Can you work these out from the model? Positions are in its coordinate system, mm. A direction names the side the tool comes from. Round coordinates to 2 decimals unless told otherwise and drop trailing zeros. Order: outer loops, then holes, each group sorted by start corner. A loop starts at its lowest first (then second) coordinate and runs counter-clockwise, first axis right, second up. Notation, with made-up numbers: (-11.5, 86) - (4.5, 86) arc R14 ccw to (4.5, 97) - close; hole circle Ø1 at (54.5, 89). An arc over 180 degrees is marked (long way). Write item = value, one per line.
from build123d import *

# Parameters (mm, degrees)
SKETCH019_W          = 124
SKETCH019_H          = 24.5
SKETCH019_R          = 2.5
PAD010_DEPTH         = 2
SKETCH018_R          = 3.175
PAD011_DEPTH         = 4.1125
PAD012_DEPTH         = 12.25
POCKET005_DEPTH      = 373.382623
POCKET005_DEPTH_BACK = 485.092667
SKETCH022_W          = 3
SKETCH022_H          = 16.275
POCKET006_DEPTH      = 14.161
POCKET006_DEPTH_BACK = 15.001


with BuildPart() as part:
    # Sketch019 → Pad010 (new body)
    with BuildSketch(Plane.XZ.offset(13)):
        with Locations((78, 0)):
            Rectangle(SKETCH019_W, SKETCH019_H)
        with Locations((30, 0)):
            Circle(SKETCH019_R, mode=Mode.SUBTRACT)
        with BuildLine():
            ThreePointArc((90.8685, 2.143), (88.7255, 0), (90.8685, -2.143))
            Line((90.8685, -2.143), (98.806, -2.143))
            ThreePointArc((98.806, -2.143), (100.949, 0), (98.806, 2.143))
            Line((98.806, 2.143), (90.8685, 2.143))
        make_face(mode=Mode.SUBTRACT)
    extrude(amount=PAD010_DEPTH)

    # Sketch018 → Pad011 (join)
    with BuildSketch(Plane.XY.offset(12.25)):
        with BuildLine():
            Line((16, -13), (10.43, -13))
            Line((10.43, -13), (10.43, 3.73))
            ThreePointArc((10.43, 3.73), (2.257465, 13.912767), (-9.45279, 8.137908))
            ThreePointArc((-26.289956, 7.402782), (-17.64833, 2.661824), (-9.45279, 8.137908))
            Line((-26.289956, 7.402782), (-13.355703, -15))
            Line((-13.355703, -15), (16, -15))
            Line((16, -15), (16, -13))
        make_face()
        with Locations((0, 3.73)):
            Circle(SKETCH018_R, mode=Mode.SUBTRACT)
    pad011 = extrude(amount=-PAD011_DEPTH)

    # Mirrored003: Pad011 across XY
    add(pad011.mirror(Plane.XY))

    # Sketch020 → Pad012 (join, symmetric)
    with BuildSketch(Plane.XY):
        Polygon((-26.289956, 7.402782), (-28.289956, 9.134833), (-14.355703, -15), (-13.355703, -15), align=None)
    extrude(amount=PAD012_DEPTH, both=True)

    # Sketch021 → Pocket005 (cut, two sides)
    with BuildSketch(Plane.YZ) as pocket005_sk:
        with BuildLine():
            ThreePointArc((-13, 12.25), (-11.749286, 10.934524), (-10, 10.45))
            Line((-10, 10.45), (14.16, 10.45))
            Line((14.16, 12.25), (14.16, 10.45))
            Line((14.16, 12.25), (-13, 12.25))
        make_face()
    pocket005 = extrude(amount=-POCKET005_DEPTH, mode=Mode.SUBTRACT) + extrude(pocket005_sk.sketch, amount=POCKET005_DEPTH_BACK, mode=Mode.SUBTRACT)

    # Mirrored004: Pocket005 across Sketch021 H_Axis
    add(pocket005.mirror(Plane.XY), mode=Mode.SUBTRACT)

    # Sketch022 → Pocket006 (cut, two sides)
    with BuildSketch(Plane.XZ) as pocket006_sk:
        with Locations((-14.855703, 0)):
            Rectangle(SKETCH022_W, SKETCH022_H)
    extrude(amount=-POCKET006_DEPTH, mode=Mode.SUBTRACT)
    extrude(pocket006_sk.sketch, amount=POCKET006_DEPTH_BACK, mode=Mode.SUBTRACT)


solid = part.part
(1) If we section it at C-C (y = -1.5): Write out the boundary of the cut face in (x, z), plus the area to 3 significant figures.
Computed:
outline = (-22.15, -10.45) - (10.43, -10.45) - (10.43, -8.14) - (-21.15, -8.14) - (-21.15, 8.14) - (10.43, 8.14) - (10.43, 10.45) - (-22.15, 10.45) - close
area = 167 mm^2
(2) On a 3-axis mill with a long thin cutter (end or side, diameter ignored), from which of +Z, -Z, +X, -X, +Y, -Y can I reach the whole of each face in a straight line? I mean faces 5 (the face through (-21.253, -1.321, 0.114)), 6 (the face through (-4, -1, -10.45)), 7 (the face through (10.43, -5, -9)). Say none if no direction works.
Computed:
face_5 = +X, +Y
face_6 = -Z, +X, -X, +Y
face_7 = +Z, -Z, +X, +Y
(3) If we section it at A-A (x = 13.5): Write out the boundary of the cut face in (y, z).
Computed:
outline = (-15, -12.25) - (-13, -12.25) - (-13, -8.14) - (-15, -8.14) - close; (-15, 8.14) - (-13, 8.14) - (-13, 12.25) - (-15, 12.25) - close
(4) If I drill on line 1 (Y direction, x = 0, z = 9.15) (3 decimals); line 2 (X direction, y = 3.73, z = -9) (3 decimals); line 3 (Y direction, x = 123.5, z = 8.5), over which ranges is the centre line in solid material (lowest first)? Write a range as from..to.
Computed:
line_1 = -15..0.555, 6.905..14.16
line_2 = -25.169..-22.457, -13.669..-3.175, 3.175..10.43
line_3 = -15..-13
(5) Will these pins go through, and if not, where does the flat tip stop? P1, Ø7, axis at x = -16, y = -2, coming from the +Z side; P2, Ø1.5, axis at y = 0, z = 4.5, coming from the -X side; P3, Ø2, axis at y = -9.5, z = -6.5, coming from the -X side; P4, Ø4, axis at x = 0, y = 3.73, coming from the -Z side.
Computed:
P1 = 10.45
P2 = -23.45
P3 = -18.11
P4 = through
(6) If we section it at D-D (x = 67.5): Write out the boundary of the cut face in (y, z), plus the area to 3 significant figures.
Computed:
outline = (-15, -12.25) - (-13, -12.25) - (-13, 12.25) - (-15, 12.25) - close
area = 49.0 mm^2
(7) If we section it at B-B (z = 0): Write out the boundary of the cut face in (x, y), plus the area to 3 significant figures.
Computed:
outline = (-28.29, 9.13) - (-16.36, -11.54) - (-16.36, -9.8) - (-26.29, 7.4) - close; (16, -15) - (27.5, -15) - (27.5, -13) - (16, -13) - close; (32.5, -15) - (88.73, -15) - (88.73, -13) - (32.5, -13) - close; (100.95, -15) - (140, -15) - (140, -13) - (100.95, -13) - close
area = 232 mm^2
(8) Thinking about a two-plate mould opening in Y: for faces 1 (the face through (-1, -3, 8.137)), 2 (the face through (2.45, 13.87, -9.31)), 3 (the face through (79, -15, 0)), 4 (the face through (-0.41, 6.88, -9.31)), which applies, +Y half, -Y half, draft (parallel to the pull), parting line (faces both ways), or undercut?
Computed:
face_1 = draft
face_2 = +Y half
face_3 = -Y half
face_4 = undercut
